Autodesk Inventor part; units mm, degrees
ref_plane "YZ Plane" through (0, 0, 0) normal (1, 0, 0) x (0, 1, 0)
ref_plane "XZ Plane" through (0, 0, 0) normal (0, 1, 0) x (-1, 0, 0)
ref_plane "XY Plane" through (0, 0, 0) normal (0, 0, 1) x (1, 0, 0)
ref_plane "Work Plane1" through (0, 3, 0) normal (0, 1, 0) x (1, 0, 0)
sketch "Sketch2" plane through (0, 3, 0) normal (0, 1, 0) x (1, 0, 0)
  line L0 (-11.25, -11.25) -> (-3.75, -11.25)
  line L1 (-3.75, -11.25) -> (-3.75, -3.75)
  line L2 (-3.75, -3.75) -> (-11.25, -3.75)
  line L3 (-11.25, -3.75) -> (-11.25, -11.25)
  line L4 (0, -15) -> (0, 0)
  line L5 (0, 0) -> (-15, 0)
  line L6 (-3.75, -11.25) -> (-2.75, -11.25)
  line L7 (-2.75, -11.25) -> (-2.75, -8.25)
  line L8 (-2.75, -8.25) -> (-3.75, -8.25)
  line L9 (-3.75, -8.25) -> (-3.75, -11.25)
  line L10 (-14.1659, -7.5) -> (-0.7229, -7.5) construction
  line L11 (-7.5, -11.25) -> (-7.5, -3.75) construction
  line L12 (-3.75, -3.75) -> (-2.75, -3.75)
  line L13 (-2.75, -3.75) -> (-2.75, -6.75)
  line L14 (-2.75, -6.75) -> (-3.75, -6.75)
  line L15 (-11.25, -11.25) -> (-12.25, -11.25)
  line L16 (-12.25, -11.25) -> (-12.25, -8.25)
  line L17 (-12.25, -8.25) -> (-11.25, -8.25)
  line L18 (-0.8341, -7.5) -> (-14.2771, -7.5) construction
  line L19 (-12.25, -3.75) -> (-12.25, -6.75)
  line L20 (-11.25, -3.75) -> (-12.25, -3.75)
  line L21 (-12.25, -6.75) -> (-11.25, -6.75)
  dimension "d4" = 7.5
  dimension "d5" = 7.5
  dimension "d6" = 3.75
  dimension "d7" = 3.75
  dimension "d8" = 3
  dimension "d9" = 1
extrude "Extrusion2" add sketch "Sketch2" along normal blind 30
ref_plane "Work Plane2" through (-12.25, 3, 11.25) normal (0, 0, 1) x (1, 0, 0)
sketch "Sketch3" plane through (-12.25, 3, 11.25) normal (0, 0, 1) x (1, 0, 0)
  line L0 (0, 30) -> (9.5, 30)
  line L1 (9.5, 30) -> (0, 30)
  line L2 (4.75, 30) -> (4.75, 36.5)
  line L3 (4.75, 36.5) -> (2.75, 36.5)
  arc A0 (2.75, 43.5578) -> (0, 30) centre (2.75, 36.5) ccw
  line L4 (0, 0) -> (0, 30)
  line L5 (0, 30) -> (0, 31.5)
  arc A1 (0.071, 41.5384) -> (0, 31.5) centre (2.75, 36.5) ccw
  line L6 (9.5, 0) -> (9.5, 30)
  line L7 (9.5, 30) -> (9.5, 31.5)
  line L8 (0.071, 41.5384) -> (-0.5634, 42.7317)
  line L9 (-0.5634, 42.7317) -> (-1.5024, 44.4976)
  arc A2 (-1.5024, 44.4976) -> (0.615, 27.6974) centre (2.75, 36.5) ccw
  arc A3 (3.4191, 47.0839) -> (0.6661, 26.1017) centre (2.75, 36.5) ccw
  line L10 (0, 30) -> (9.5, 30)
  line L11 (9.5, 31.5) -> (0, 31.5)
  line L12 (0.615, 27.6974) -> (8.885, 27.6974)
  line L13 (9.2653, 26.1017) -> (0.6661, 26.1017)
  line L14 (4.75, 36.5) -> (4.75, 49.394)
  line L15 (-1.5024, 44.4976) -> (-2.2288, 45.8637)
  arc A4 (2.75, 42.2064) -> (0.071, 41.5384) centre (2.75, 36.5) ccw
  line L16 (2.75, 42.2064) -> (2.75, 47.105)
  line L17 (4.75, 49.394) -> (4.75, 23.6593)
  line L18 (4.75, 36.5) -> (6.75, 36.5)
  arc A5 (9.5, 30) -> (6.75, 43.5578) centre (6.75, 36.5) ccw
  line L19 (9.5, 30) -> (9.5, 31.5)
  arc A6 (9.5, 31.5) -> (9.429, 41.5384) centre (6.75, 36.5) ccw
  line L20 (9.429, 41.5384) -> (10.0634, 42.7317)
  line L21 (10.0634, 42.7317) -> (11.0024, 44.4976)
  arc A7 (8.885, 27.6974) -> (11.0024, 44.4976) centre (6.75, 36.5) ccw
  arc A8 (8.8339, 26.1017) -> (6.0809, 47.0839) centre (6.75, 36.5) ccw
  line L22 (11.0024, 44.4976) -> (11.7288, 45.8637)
  arc A9 (9.429, 41.5384) -> (6.75, 42.2064) centre (6.75, 36.5) ccw
  line L23 (6.75, 42.2064) -> (6.75, 47.105)
  line L24 (6.75, 47.105) -> (2.75, 47.105)
  line L25 (2.75, 42.2064) -> (6.75, 42.2064)
  point P0 (12.25, -3)
  point P1 (0, 27.8698)
  point P2 (4.75, 42.947)
  point P3 (9.5, 27.8698)
  point P4 (0, 26.2577)
  point P5 (9.5, 26.2577)
  dimension "d28" = 6.5
  dimension "d29" = 2
  dimension "d31" = 1.5
  dimension "d33" = 2
  dimension "d34" = 1.3514
  dimension "d59" = 28
  dimension "d60" = 1.5473
extrude "Extrusion5" add sketch "Sketch3" against normal blind 7.5 contours L5 L11 L2 L0 | A0 L8 A1 L5 | L2 L11 L7 L0 | L9 L15 A3 L16 A0 | A0 L16 A4 L8 | L4 A3 L15 A2 | L7 A6 L20 A5 | A7 L22 A8 L6 | L20 A9 L23 A5 | A5 L23 A8 L22 L21
extrude "Extrusion6" cut sketch "Sketch3" against normal blind 7.5 contours L0 L17 L12 A2 L4 | L0 L6 A7 L12 L17
sketch "Sketch4" plane through (-2.75, 3, 3.75) normal (0, 0, -1) x (-1, 0, 0)
  line L0 (9.5, 0) -> (0, 0)
  line L1 (3.75, 0) -> (5.75, 0)
  line L2 (5.75, 0) -> (5.75, 5)
  line L3 (5.75, 5) -> (3.75, 5)
  line L4 (3.75, 5) -> (3.75, 0)
  line L5 (9.5, 0) -> (9.5, 26.2577)
  line L6 (1, 0) -> (1, 27.6974)
  line L7 (3.75, 5) -> (1, 5)
  line L8 (1, 3.5) -> (3.75, 3.5)
  line L9 (3.75, 3.5) -> (3.75, 5)
  line L10 (4.75, 0) -> (4.75, 5)
  line L11 (0, 0) -> (9.5, 0)
  line L12 (5.75, 0) -> (3.75, 0)
  line L13 (3.75, 5) -> (5.75, 5)
  line L14 (5.75, 5) -> (5.75, 0)
  line L15 (5.75, 5) -> (8.5, 5)
  line L16 (8.5, 3.5) -> (5.75, 3.5)
  line L17 (5.75, 3.5) -> (5.75, 5)
  line L18 (1, 3.5) -> (1, 5)
  line L19 (8.5, 3.5) -> (8.5, 5)
  point P0 (-2.75, -3)
  point P1 (5.75, 0)
  point P2 (5.75, 3.5)
  point P3 (3.75, 3.5)
  dimension "d62" = 2
  dimension "d63" = 4.75
  dimension "d64" = 5
  dimension "d65" = 1.5
extrude "Extrusion7" cut sketch "Sketch4" against normal through all contours L0 L10 L3 L2 | L0 L4 L3 L10 | L2 L15 L19 L16 | L8 L6 L7 L4
extrude "Extrusion8" add sketch "Sketch3" against normal blind 2 contours L4 A2 L9 A0 | L0 L17 L12 A2 L4 | L0 L6 A7 L12 L17 | A1 A4 L25 L14 L2 L11 | A5 L21 A7 L6 | L2 L14 L25 A9 A6 L11 | L16 L24 L14 L25 | L23 L25 L14 L24
properties part number "SlangHållare"
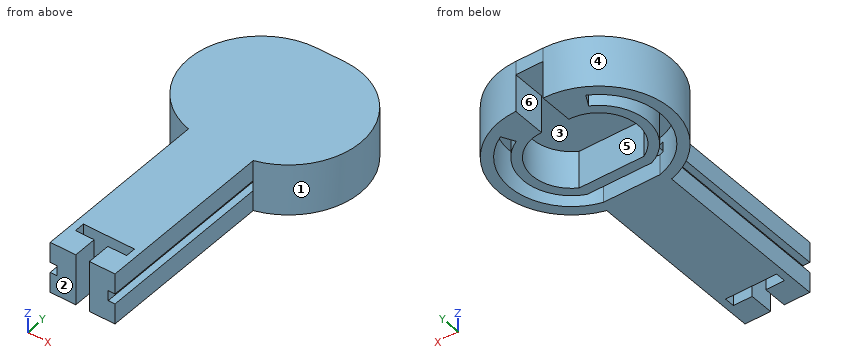
Model file for the job. Use its own axes, mm. Face numbers are marked on the shaded views. A direction names the side the tool comes from. Give positions to 0.01 mm unless a question says otherwise; leave off trailing zeros. Loops run counter-clockwise (first coordinate to the right, second up) from the corner with the lowest first, then second, coordinate; pieces in that order, holes last.
1) Saw through at A-A (x = -9). Write the cut outline in (y, z) (3 decimals), plus the area to 3 significant figures.
2) Pull direction Y, two halves, no side cores. Call the marked faces 1, 2 and 3: +Y half, -Y half, draft (parallel to the pull), parting line (faces both ways), or undercut.
3) Saw through at B-B (z = 10). Write the cut outline in (x, y) (3 decimals), plus the area to 3 significant figures.
4) Saw through at C-C (y = 15.5). Write the cut outline in (x, z).
5) Flat gauge pins, fed straight in: pin 1 Ø0.8 at (y, z) = (7.5, 9.5) entering from +X; pin 2 Ø0.8 at (y, z) = (30.5, 7) entering from -X; pin 3 Ø1.2 at (y, z) = (30.5, 7) entering from +X. Where does each tip first touch, or does it go through?
6) Tool access for the marked faces 4, 5 and 6: list every direction of +Z, -Z, +X, -X, +Y, -Y with a clear straight run to the whole face (end or side of a thin tool).
7) Wall check: line 1 (Y direction, x = -4.75, z = 8.5); line 2 (X direction, y = 7.5, z = 10.5); line 3 (X direction, y = 33.5, z = 7). Give the ranges that are in metal, low to high.
8) Saw through at D-D (z = 5.5). Write the cut outline in (x, y) (3 decimals).
Answer block:
1. outline: (3, 3.75) - (6.5, 3.75) - (6.5, 11.25) - (3, 11.25) - close; (8, 3.75) - (30.697, 3.75) - (30.697, 9.25) - (33, 9.25) - (33, 3.75) - (34.5, 3.75) - (34.5, 9.25) - (50.105, 9.25) - (50.105, 11.25) - (8, 11.25) - close
1. area: 244 mm2
2. face 1: parting line
2. face 2: -Y half
2. face 3: undercut
3. outline: (-12.25, 3) - (-8.5, 3) - (-8.5, 6.5) - (-11.25, 6.5) - (-11.25, 8) - (-3.75, 8) - (-3.75, 6.5) - (-6.5, 6.5) - (-6.5, 3) - (-2.75, 3) - (-2.75, 29.258) arc R10.605 ccw to (-5.5, 50.105) - (-9.5, 50.105) arc R10.605 ccw to (-12.25, 29.258) - close
3. area: 667 mm2
4. outline: (-12.25, 3.75) - (-2.75, 3.75) - (-2.75, 6.75) - (-3.75, 6.75) - (-3.75, 8.25) - (-2.75, 8.25) - (-2.75, 11.25) - (-12.25, 11.25) - (-12.25, 8.25) - (-11.25, 8.25) - (-11.25, 6.75) - (-12.25, 6.75) - close
5. pin 1: stops at x = -2.75
5. pin 2: stops at x = -15.71
5. pin 3: stops at x = 0.97
6. face 4: +Z, -Z, -X
6. face 5: -Z
6. face 6: -Z, +Y
7. line 1: y = 3 to 6.5, 8 to 30.7, 33 to 34.5, 45.16 to 50.08
7. line 2: x = -12.25 to -11.25, -3.75 to -2.75
7. line 3: x = -18.24 to -16.29, -13.22 to -1.78, 1.29 to 3.24
8. outline: (-12.25, 3) - (-8.5, 3) - (-8.5, 6.5) - (-11.25, 6.5) - (-11.25, 8) - (-3.75, 8) - (-3.75, 6.5) - (-6.5, 6.5) - (-6.5, 3) - (-2.75, 3) - (-2.75, 29.258) arc R10.605 ccw to (-5.5, 50.105) - (-5.5, 45.206) arc R5.707 cw to (-2.821, 44.538) arc R5.706 cw to (-2.75, 34.5) - (-12.25, 34.5) arc R5.706 cw to (-12.179, 44.538) arc R5.706 cw to (-9.5, 45.206) - (-9.5, 50.105) arc R10.605 ccw to (-12.25, 29.258) - close; hole (-13.752, 47.498) arc R9.058 ccw to (-11.635, 30.697) - (-3.365, 30.697) arc R9.058 ccw to (-1.248, 47.498) - (-2.187, 45.732) arc R7.058 cw to (-2.75, 33) - (-12.25, 33) arc R7.058 cw to (-12.813, 45.732) - close
